Input: dimensioned drawing with shaded views. Units: mm. Origin: part minimum x, y, z. Round coordinates to 2 decimals unless told otherwise and drop trailing zeros. Write each loop counter-clockwise with the first axis right and the second up, starting at its lowest first coordinate (ties: lowest second). Pieces come first, ordered by that corner, then holes. Notation, with made-up numbers: (20, 85) - (54, 85) arc R23 cw to (54, 121) - close; hole circle Ø10 at (0.5, 34). An arc over 180 degrees is marked (long way). Write item = value, one per line. Start each with the question number.
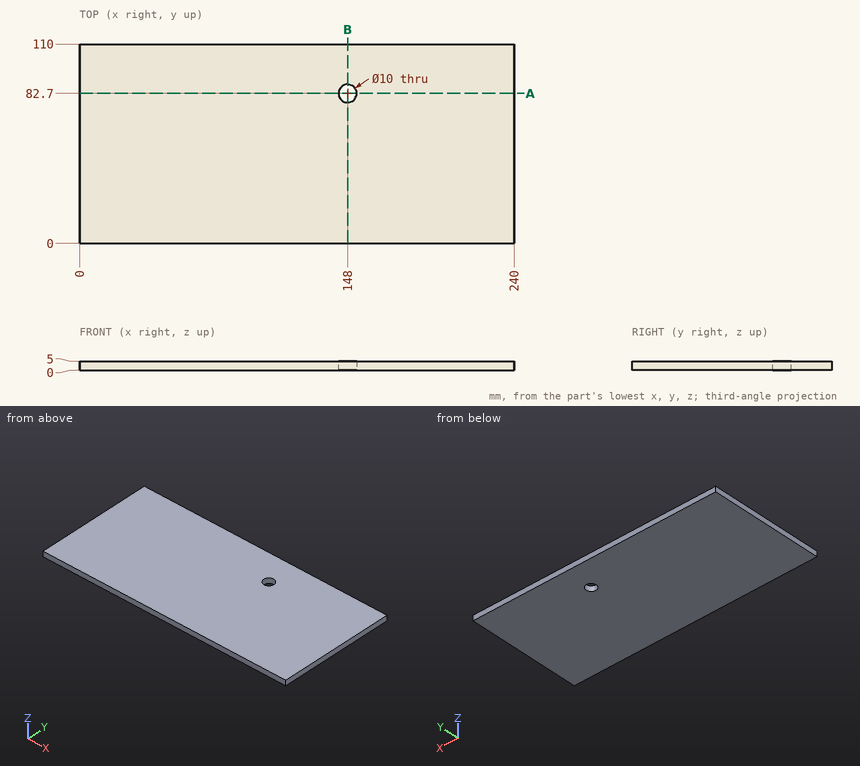
(1) Ray query, L1, parallel to Y at x = 148, z = 1.1; L2, parallel to X at y = 87, z = 3.7; L3, parallel to X at y = 78.5, z = 3.7. Return the intervals inside material, ascending. Write a range as from..to.
(2) Section A-A (y = 82.7). Return the cut outline in (x, z), plus the area to 3 significant figures.
(3) Contact query for flat-ended pins moving along their axis: P1, Ø1.5, axis at x = 44.5, z = 1, coming from the -Y side; P2, Ø8, axis at x = 148, y = 82.7, coming from the -Z side. Output: stop coordinate, or through.
(4) Section B-B (x = 148). Return the cut outline in (y, z), plus the area to 3 significant figures.
Solution:
q1.L1 = 0..77.7, 87.7..110
q1.L2 = 0..145.45, 150.55..240
q1.L3 = 0..145.29, 150.71..240
q2.outline = (0, 0) - (143, 0) - (143, 5) - (0, 5) - close; (153, 0) - (240, 0) - (240, 5) - (153, 5) - close
q2.area = 1,150 mm^2
q3.P1 = 0
q3.P2 = through
q4.outline = (0, 0) - (77.7, 0) - (77.7, 5) - (0, 5) - close; (87.7, 0) - (110, 0) - (110, 5) - (87.7, 5) - close
q4.area = 500 mm^2
